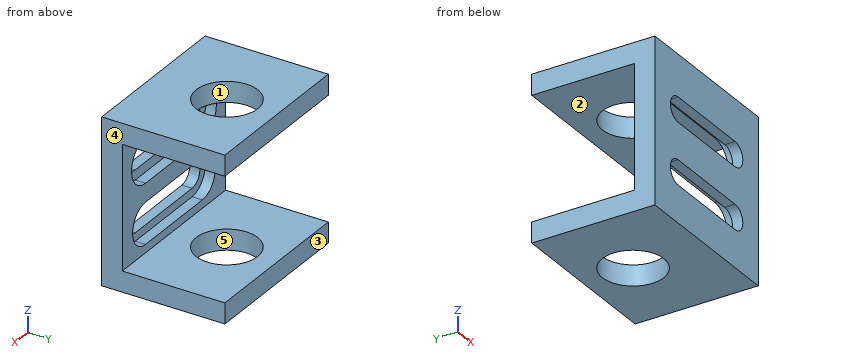
from build123d import *

# Parameters (mm, degrees)
BOSS_EXTRUDE2_DEPTH = 25.4
SKETCH3_R           = 4.7625
CUT_EXTRUDE1_DEPTH  = 36.576
CUT_EXTRUDE2_DEPTH  = 66.04
CUT_EXTRUDE3_DEPTH  = 1.5875
CUT_EXTRUDE4_DEPTH  = 1.5875
CUT_EXTRUDE5_DEPTH  = 45.510676996


with BuildPart() as part:
    # Sketch1 → Boss-Extrude2 (new body)
    with BuildSketch(Plane(origin=(-35.145897579, 0, 0), x_dir=(0, 0, -1), z_dir=(1, 0, 0))):
        Polygon((0, 0), (-19.05, 0), (-22.225, 0), (-22.225, 19.05), (-19.05, 19.05), (-19.05, 3.175), (0, 3.175), (0, 19.05), (3.175, 19.05), (3.175, 0), align=None)
    extrude(amount=BOSS_EXTRUDE2_DEPTH)

    # Sketch3 → Cut-Extrude1 (cut)
    with BuildSketch(Plane(origin=(0, 0, -3.175), x_dir=(-1, 0, 0), z_dir=(0, 0, -1))):
        with Locations((22.445897579, 11.3665)):
            Circle(SKETCH3_R)
    extrude(amount=-CUT_EXTRUDE1_DEPTH, mode=Mode.SUBTRACT)

    # Sketch4 → Cut-Extrude2 (cut)
    with BuildSketch(Plane(origin=(0, 3.175, 0), x_dir=(1, 0, 0), z_dir=(0, 1, 0))):
        with BuildLine():
            Line((-29.430897579, -2.54), (-15.460897579, -2.54))
            ThreePointArc((-15.460897579, -2.54), (-13.555897579, -4.445), (-15.460897579, -6.35))
            Line((-15.460897579, -6.35), (-29.430897579, -6.35))
            ThreePointArc((-29.430897579, -6.35), (-31.335897579, -4.445), (-29.430897579, -2.54))
        make_face()
    extrude(amount=-CUT_EXTRUDE2_DEPTH, mode=Mode.SUBTRACT)

    # Sketch7 → Cut-Extrude3 (cut)
    with BuildSketch(Plane(origin=(0, 3.175, 0), x_dir=(1, 0, 0), z_dir=(0, 1, 0))):
        with BuildLine():
            Line((-29.430897579, -1.27), (-15.460897579, -1.27))
            ThreePointArc((-15.460897579, -1.27), (-12.285897579, -4.445), (-15.460897579, -7.62))
            Line((-15.460897579, -7.62), (-29.430897579, -7.62))
            ThreePointArc((-29.430897579, -7.62), (-32.605897579, -4.445), (-29.430897579, -1.27))
        make_face()
    extrude(amount=-CUT_EXTRUDE3_DEPTH, mode=Mode.SUBTRACT)

    # Sketch8 → Cut-Extrude4 (cut)
    # profile 1 of 2: a face of its own
    with BuildSketch(Plane(origin=(0, 3.175, 0), x_dir=(1, 0, 0), z_dir=(0, 1, 0))):
        with BuildLine():
            Line((-15.460897579, -17.327840803), (-29.430897579, -17.327840803))
            ThreePointArc((-29.430897579, -17.327840803), (-32.859897579, -13.898840803), (-29.430897579, -10.469840803))
            Line((-29.430897579, -10.469840803), (-15.460897579, -10.469840803))
            ThreePointArc((-15.460897579, -10.469840803), (-12.031897579, -13.898840803), (-15.460897579, -17.327840803))
        make_face()
        with BuildLine():
            ThreePointArc((-29.430897579, -11.993840803), (-31.335897579, -13.898840803), (-29.430897579, -15.803840803))
            Line((-29.430897579, -15.803840803), (-15.460897579, -15.803840803))
            ThreePointArc((-15.460897579, -15.803840803), (-13.555897579, -13.898840803), (-15.460897579, -11.993840803))
            Line((-15.460897579, -11.993840803), (-29.430897579, -11.993840803))
        make_face(mode=Mode.SUBTRACT)
    # profile 2 of 2: a face of its own
    with BuildSketch(Plane(origin=(0, 3.175, 0), x_dir=(1, 0, 0), z_dir=(0, 1, 0))):
        with BuildLine():
            Line((-29.430897579, -11.993840803), (-15.460897579, -11.993840803))
            ThreePointArc((-15.460897579, -11.993840803), (-13.555897579, -13.898840803), (-15.460897579, -15.803840803))
            Line((-15.460897579, -15.803840803), (-29.430897579, -15.803840803))
            ThreePointArc((-29.430897579, -15.803840803), (-31.335897579, -13.898840803), (-29.430897579, -11.993840803))
        make_face()
    extrude(amount=-CUT_EXTRUDE4_DEPTH, mode=Mode.SUBTRACT)

    # Sketch8_3 → Cut-Extrude5 (cut, through all)
    with BuildSketch(Plane(origin=(0, 3.175, 0), x_dir=(1, 0, 0), z_dir=(0, 1, 0))):
        with BuildLine():
            Line((-29.430897579, -11.993840803), (-15.460897579, -11.993840803))
            ThreePointArc((-15.460897579, -11.993840803), (-13.555897579, -13.898840803), (-15.460897579, -15.803840803))
            Line((-15.460897579, -15.803840803), (-29.430897579, -15.803840803))
            ThreePointArc((-29.430897579, -15.803840803), (-31.335897579, -13.898840803), (-29.430897579, -11.993840803))
        make_face()
    extrude(amount=-CUT_EXTRUDE5_DEPTH, mode=Mode.SUBTRACT)


solid = part.part
Geometry: final body of the model. Coordinates: model frame, mm. Face numbers are marked on the shaded views. A direction names the side the tool comes from. Give positions to 0.01 mm unless a question says otherwise; leave off trailing zeros. Write each loop counter-clockwise with the first axis right and the second up, starting at its lowest first coordinate (ties: lowest second). Pieces come first, ordered by that corner, then holes. Notation, with made-up numbers: (-28, -11) -> (-15, -11) arc R26 cw to (-15, 28) -> close; hole circle Ø3 at (53.5, 43). An arc over 180 degrees is marked (long way). Answer in a Markdown table with one row per item.
(1) Section query D-D on y = 16.75. Return loops of the section in (x, z) (3 decimals), then the cut area to 3 significant figures.
Answers below:
| item | result |
|---|---|
| outline | (-35.146, -3.175) -> (-9.746, -3.175) -> (-9.746, 0) -> (-35.146, 0) -> close; (-35.146, 19.05) -> (-9.746, 19.05) -> (-9.746, 22.225) -> (-35.146, 22.225) -> close |
| area | 161 mm^2 |
(2) Section query A-A on y = 2. Return loops of the section in (x, z) (3 decimals), then the cut area to 3 significant figures.
Answers below:
| item | result |
|---|---|
| outline | (-35.146, -3.175) -> (-9.746, -3.175) -> (-9.746, 22.225) -> (-35.146, 22.225) -> close; hole (-29.431, 1.27) -> (-15.461, 1.27) arc R3.175 ccw to (-15.461, 7.62) -> (-29.431, 7.62) arc R3.175 ccw to start; hole (-29.431, 10.47) -> (-15.461, 10.47) arc R3.429 ccw to (-15.461, 17.328) -> (-29.431, 17.328) arc R3.429 ccw to start |
| area | 392 mm^2 |
(3) Draft query along X for the marked faces 3, 4 and 5. Return one class per face: +X half, -X half, draft (parallel to the pull), parting line (faces both ways), or undercut.
Answers below:
| item | result |
|---|---|
| face 3 | draft |
| face 4 | +X half |
| face 5 | undercut |
(4) Section query C-C on z = 14.25. Return loops of the section in (x, y) (1 decimal).
Answers below:
| item | result |
|---|---|
| outline | (-35.1, 0) -> (-31.3, 0) -> (-31.3, 1.6) -> (-32.8, 1.6) -> (-32.8, 3.2) -> (-35.1, 3.2) -> close; (-13.6, 0) -> (-9.7, 0) -> (-9.7, 3.2) -> (-12, 3.2) -> (-12, 1.6) -> (-13.6, 1.6) -> close |
(5) Set-up query: the marked faces 1 and 2. Return all of +Z, -Z, +X, -X, +Y, -Y with unobstructed straight access to the full face (end or side cutting, diameter ignored); none if empty.
Answers below:
| item | result |
|---|---|
| face 1 | +Z, -Z |
| face 2 | +X, -X, +Y |
(6) Pin query (flat end, axial travel): pin 1 (2 mm diameter, centred on x = -27.5, z = 14.5, fed in from +Y); pin 2 (10 mm diameter, centred on x = -24.5, z = 3, fed in from +Y); pin 3 (5.5 mm diameter, centred on x = -16.5, z = 11, fed in from +Y) (3 decimals); pin 4 (3 mm diameter, centred on x = -21.5, z = 5, fed in from +Y). Return the tip coordinate at first contact, or that it passes through.
Answers below:
| item | result |
|---|---|
| pin 1 | through |
| pin 2 | y = 19.05 |
| pin 3 | y = 3.175 |
| pin 4 | y = 1.59 |
(7) Section query B-B on x = -23.5. State how many separate pieces and enclosed holes the cut face has, then the cut area to 3 significant figures.
Answers below:
| item | result |
|---|---|
| separate pieces | 5 |
| enclosed holes | 0 |
| area | 89.4 mm^2 |
(8) Ray query, line 1 along Z through (x, y) = (-16.5, 1.25) (3 decimals); line 2 along Z through (x, y) = (-22.75, 17.5) (3 decimals); line 3 along Y through (x, z) = (-14.75, 0.5) (3 decimals). Return the intervals inside material, ascending. Write a range as [from, to].
Answers below:
| item | result |
|---|---|
| line 1 | [-3.175, 2.54], [6.35, 11.994], [15.804, 22.225] |
| line 2 | [-3.175, 0], [19.05, 22.225] |
| line 3 | [0, 3.175] |
